Check sheet for the modelled part. Datum: model origin and axes. Units: mm. Face numbers are marked on the shaded views. A direction names the side the tool comes from. Coordinates: 2 decimals unless noted, no trailing zeros. Order: outer loops, then holes, each group sorted by start corner. A loop starts at its lowest first (then second) coordinate and runs counter-clockwise, first axis right, second up.
1. Set-up check for the marked faces 1, 2, 3 and 4: record each of +Z, -Z, +X, -X, +Y, -Y from which the full face is reachable in a straight line by a thin tool's end or side.
2. Cross-section at A-A (z = 0). Enter the section's corners in (x, y) (3 decimals), then the cut area to 3 significant figures.
3. Cross-section at D-D (y = -4.75). Enter the section's corners in (x, z), then the cut area to 3 significant figures.
4. Cross-section at C-C (x = 13.5). Enter the section's corners in (y, z).
5. Thickness scan on line 1 (X direction, y = 0, z = 4); line 2 (X direction, y = -12, z = -4); line 3 (X direction, y = -5.5, z = 10.5). Record the ranges inside material, lowest first.
6. Gauge pin test, flat ends, axial feed: pin 1 Ø10 at (y, z) = (-8.5, 10) entering from -X; pin 2 Ø2 at (x, z) = (13, -9) entering from -Y; pin 3 Ø8 at (x, z) = (4, 7) entering from +Y; pin 4 Ø3 at (x, z) = (13.5, 0) entering from +Y. Record the tip position at first contact, or that the pin passes through.
7. Draft check along X on the marked faces 5, 6 and 7. Enter one of: released by +X, released by -X, zero draft, split by the parting line, or undercut.
8. Cross-section at B-B (y = 0). Enter the section's corners in (x, z) (3 decimals).
```python
from build123d import *

# Parameters (mm, degrees)
CUT_EXTRUDE1_REACH      = 28.096
CUT_EXTRUDE1_END_RADIUS = 9
SKETCH2_R               = 2
CIRPATTERN1_COUNT       = 2
CIRPATTERN1_ANGLE       = 90


with BuildPart() as part:
    # Sketch1 → Revolve1 (revolve)
    with BuildSketch(Plane.XY, mode=Mode.PRIVATE) as revolve1_sk:
        Polygon((0, 2.5), (17, 2.5), (17, 9), (10, 9), (10, 14), (8.5, 14), (8.5, 12.475), (1.5, 12.475), (1.5, 14), (0, 14), align=None)
    revolve(revolve1_sk.sketch.rotate(Axis((17.85, 0, 0), (-1, 0, 0)), 90), axis=Axis((17.85, 0, 0), (-1, 0, 0)))

    # Cut-Extrude1: up to this cylinder (the profile starts inside it)
    cut_extrude1_end = Plane(origin=(13.5, 0, 0), z_dir=(1, 0, 0)) * Cylinder(CUT_EXTRUDE1_END_RADIUS, 75.192, mode=Mode.PRIVATE)
    # Sketch2 → Cut-Extrude1 (cut, up to the surface)
    with BuildSketch(Plane(origin=(0, 0, 0), x_dir=(1, 0, 0), z_dir=(0, 1, 0)), mode=Mode.PRIVATE) as cut_extrude1_sk1:
        with Locations(Location((13.5, 0, 0), (0, 0, 270))):
            Circle(SKETCH2_R)
    cut_extrude1_tool1 = extrude(cut_extrude1_sk1.sketch, amount=-CUT_EXTRUDE1_REACH, mode=Mode.PRIVATE) & cut_extrude1_end
    cut_extrude1 = cut_extrude1_tool1.solids().sort_by_distance((13.5, 0, 0))[0]
    add(cut_extrude1, mode=Mode.SUBTRACT)

    # CirPattern1: Cut-Extrude1 ×2 about axis
    cirpattern1_axis = Axis((17.85, 0, 0), (-1, 0, 0))
    for i in range(1, CIRPATTERN1_COUNT):
        add(cut_extrude1.rotate(cirpattern1_axis, i * CIRPATTERN1_ANGLE / (CIRPATTERN1_COUNT - 1)), mode=Mode.SUBTRACT)


solid = part.part
```
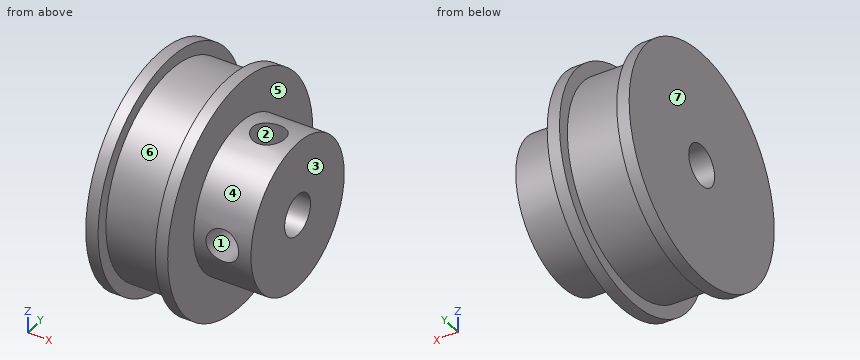
Data:
1. face 1: -Y
1. face 2: +Z
1. face 3: +Z, -Z, +X, +Y, -Y
1. face 4: +X
2. outline: (0, -14) - (1.5, -14) - (1.5, -12.475) - (8.5, -12.475) - (8.5, -14) - (10, -14) - (10, -9) - (11.5, -9) - (11.5, -2.5) - (0, -2.5) - close; (0, 2.5) - (17, 2.5) - (17, 9) - (10, 9) - (10, 14) - (8.5, 14) - (8.5, 12.475) - (1.5, 12.475) - (1.5, 14) - (0, 14) - close; (15.5, -9) - (17, -9) - (17, -2.5) - (15.5, -2.5) - close
2. area: 274 mm2
3. outline: (0, -13.17) - (1.5, -13.17) - (1.5, -11.54) - (8.5, -11.54) - (8.5, -13.17) - (10, -13.17) - (10, -7.64) - (17, -7.64) - (17, 7.64) - (10, 7.64) - (10, 13.17) - (8.5, 13.17) - (8.5, 11.54) - (1.5, 11.54) - (1.5, 13.17) - (0, 13.17) - close; hole circle Ø4 at (13.5, 0)
3. area: 335 mm2
4. outline: (-8.77, -2) arc R9 ccw (long way) to (2, 8.77) - (2, 1.5) arc R2.5 cw to (-1.5, -2) - close; (-8.77, 2) - (-2, 2) - (-2, 8.77) arc R9 ccw to start
5. line 1: x = 0 to 11.5, 15.5 to 17
5. line 2: x = 0 to 1.5, 8.5 to 10
5. line 3: x = 0 to 10
6. pin 1: stops at x = 0
6. pin 2: stops at y = -4.12
6. pin 3: stops at y = 13.45
6. pin 4: stops at y = 9
7. face 5: released by +X
7. face 6: undercut
7. face 7: released by -X
8. outline: (0, -14) - (1.5, -14) - (1.5, -12.475) - (8.5, -12.475) - (8.5, -14) - (10, -14) - (10, -9) - (17, -9) - (17, -2.5) - (0, -2.5) - close; (0, 2.5) - (11.5, 2.5) - (11.5, 9) - (10, 9) - (10, 14) - (8.5, 14) - (8.5, 12.475) - (1.5, 12.475) - (1.5, 14) - (0, 14) - close; (15.5, 2.5) - (17, 2.5) - (17, 9) - (15.5, 9) - close
